```python
from build123d import *

# Parameters (mm, degrees)
SKETCH_1_W          = 12
SKETCH_1_H          = 10
EXTRUDE_1_DEPTH     = 0.8
CUT_EXTRUDE_1_REACH = 9.851
SKETCH_2_R          = 1.5
SKETCH_2_R_2        = 0.75
SKETCH_2_R_3        = 0.375
FILLET_1_R          = 1
SKETCH_5_R          = 0.5
CUT_EXTRUDE_2_DEPTH = 8.851114571
EXTRUDE_START       = 1
SKETCH_14_R         = 2
SKETCH_14_R_2       = 1.5
EXTRUDE_2_DEPTH     = 1


with BuildPart() as part:
    # Эскиз1 → Бобышка-Вытянуть1 (new body)
    with BuildSketch(Plane.XY):
        Rectangle(SKETCH_1_W, SKETCH_1_H)
    extrude(amount=EXTRUDE_1_DEPTH)

    # Эскиз2 → Вырез-Вытянуть1 (cut, up to next)
    with BuildSketch(Plane.XY.offset(0.8), mode=Mode.PRIVATE) as cut_extrude_1_sk1:
        Circle(SKETCH_2_R)
    cut_extrude_1_tool1 = extrude(cut_extrude_1_sk1.sketch, amount=-CUT_EXTRUDE_1_REACH, mode=Mode.PRIVATE) & part.part
    # Эскиз2 → Вырез-Вытянуть1 (cut, up to next)
    with BuildSketch(Plane.XY.offset(0.8), mode=Mode.PRIVATE) as cut_extrude_1_sk2:
        with Locations((-3.6, -3)):
            Circle(SKETCH_2_R_2)
    cut_extrude_1_tool2 = extrude(cut_extrude_1_sk2.sketch, amount=-CUT_EXTRUDE_1_REACH, mode=Mode.PRIVATE) & part.part
    # Эскиз2 → Вырез-Вытянуть1 (cut, up to next)
    with BuildSketch(Plane.XY.offset(0.8), mode=Mode.PRIVATE) as cut_extrude_1_sk3:
        with Locations((3.6, 3)):
            Circle(SKETCH_2_R_2)
    cut_extrude_1_tool3 = extrude(cut_extrude_1_sk3.sketch, amount=-CUT_EXTRUDE_1_REACH, mode=Mode.PRIVATE) & part.part
    # Эскиз2 → Вырез-Вытянуть1 (cut, up to next)
    with BuildSketch(Plane.XY.offset(0.8), mode=Mode.PRIVATE) as cut_extrude_1_sk4:
        with Locations((3.25, -2)):
            Circle(SKETCH_2_R_3)
    cut_extrude_1_tool4 = extrude(cut_extrude_1_sk4.sketch, amount=-CUT_EXTRUDE_1_REACH, mode=Mode.PRIVATE) & part.part
    # Эскиз2 → Вырез-Вытянуть1 (cut, up to next)
    with BuildSketch(Plane.XY.offset(0.8), mode=Mode.PRIVATE) as cut_extrude_1_sk5:
        with Locations((-3.25, 2)):
            Circle(SKETCH_2_R_3)
    cut_extrude_1_tool5 = extrude(cut_extrude_1_sk5.sketch, amount=-CUT_EXTRUDE_1_REACH, mode=Mode.PRIVATE) & part.part
    add(cut_extrude_1_tool1.solids().sort_by_distance((0, 0, 0.8))[0], mode=Mode.SUBTRACT)
    add(cut_extrude_1_tool2.solids().sort_by_distance((-3.6, -3, 0.8))[0], mode=Mode.SUBTRACT)
    add(cut_extrude_1_tool3.solids().sort_by_distance((3.6, 3, 0.8))[0], mode=Mode.SUBTRACT)
    add(cut_extrude_1_tool4.solids().sort_by_distance((3.25, -2, 0.8))[0], mode=Mode.SUBTRACT)
    add(cut_extrude_1_tool5.solids().sort_by_distance((-3.25, 2, 0.8))[0], mode=Mode.SUBTRACT)

    # Скругление1
    fillet_1_edges = [part.edges().sort_by_distance(p)[0] for p in [
        (6, -5, 0.4),
        (-6, -5, 0.4),
        (-6, 5, 0.4),
        (6, 5, 0.4),
    ]]
    fillet(fillet_1_edges, radius=FILLET_1_R)

    # Эскиз5 → Вырез-Вытянуть2 (cut, through all)
    with BuildSketch(Plane.XY.offset(0.8)):
        with Locations((5, 0)):
            Circle(SKETCH_5_R)
        with Locations((-5, 0)):
            Circle(SKETCH_5_R)
    extrude(amount=-CUT_EXTRUDE_2_DEPTH, mode=Mode.SUBTRACT)

    # Эскиз14 → Бобышка-Вытянуть2 (add)
    with BuildSketch(Plane.XY.offset(0.8).offset(EXTRUDE_START)):
        with Locations(Location((0, 0, 0), (0, 0, 180))):
            Circle(SKETCH_14_R)
        Circle(SKETCH_14_R_2, mode=Mode.SUBTRACT)
    extrude(amount=-EXTRUDE_2_DEPTH)


solid = part.part
```
The model under review builds one solid part; all positions refer to its coordinate system, in mm. A direction names the side the tool comes from. Give positions to 0.01 mm unless a question says otherwise; leave off trailing zeros. Write each loop counter-clockwise with the first axis right and the second up, starting at its lowest first coordinate (ties: lowest second). Pieces come first, ordered by that corner, then holes. Notation, with made-up numbers: (-34.75, 9.25) -> (22.25, 9.25) arc R21 ccw to (22.25, 35.25) -> close; hole circle Ø3 at (16, 75.5). An arc over 180 degrees is marked (long way). Answer in a Markdown table with one row per item.
1) Add section C-C on z = 0.5. State the section outline as (x, y) points (3 decimals).
Worked answers:
| item | result |
|---|---|
| outline | (-6, -4) arc R1 ccw to (-5, -5) -> (5, -5) arc R1 ccw to (6, -4) -> (6, 4) arc R1 ccw to (5, 5) -> (-5, 5) arc R1 ccw to (-6, 4) -> close; hole circle Ø1 at (-5, 0); hole circle Ø1.5 at (-3.6, -3); hole circle Ø0.75 at (-3.25, 2); hole circle Ø3 at (0, 0); hole circle Ø1.5 at (3.6, 3); hole circle Ø0.75 at (3.25, -2); hole circle Ø1 at (5, 0) |
2) Clearance check with a flat-ended pin moving along its axis: P1, Ø0.9, axis at x = -3.6, y = -3, coming from the +Z side. State where the tip first meets the part, or that it passes through.
Worked answers:
| item | result |
|---|---|
| P1 | through |
3) Add section B-B on y = 3. State the section outline as (x, z) points.
Worked answers:
| item | result |
|---|---|
| outline | (-6, 0) -> (2.85, 0) -> (2.85, 0.8) -> (-6, 0.8) -> close; (4.35, 0) -> (6, 0) -> (6, 0.8) -> (4.35, 0.8) -> close |
4) Add section D-D on y = 0.25. State the section outline as (x, z) points, plus the area to 3 significant figures.
Worked answers:
| item | result |
|---|---|
| outline | (-6, 0) -> (-5.43, 0) -> (-5.43, 0.8) -> (-6, 0.8) -> close; (-4.57, 0) -> (-1.48, 0) -> (-1.48, 1.8) -> (-1.98, 1.8) -> (-1.98, 0.8) -> (-4.57, 0.8) -> close; (1.48, 0) -> (4.57, 0) -> (4.57, 0.8) -> (1.98, 0.8) -> (1.98, 1.8) -> (1.48, 1.8) -> close; (5.43, 0) -> (6, 0) -> (6, 0.8) -> (5.43, 0.8) -> close |
| area | 6.86 mm² |
5) For L1, parallel to Y at x = 0, z = 0.85; L2, parallel to Z at x = -3, y = -2.25; L3, parallel to Y at x = -3.25, z = 0.5 (3 decimals), list the stretches that pass through material, from the lowest coordinate up. Write a range as [from, to].
Worked answers:
| item | result |
|---|---|
| L1 | [-2, -1.5], [1.5, 2] |
| L2 | [0, 0.8] |
| L3 | [-5, -3.663], [-2.337, 1.625], [2.375, 5] |
6) Tool access review of faces 4 (the cylindrical face through (0, 2, 1)), 5 (the cylindrical face through (-5.715, -4.699, 0.406)): name each direction out of +Z, -Z, +X, -X, +Y, -Y from which nothing blocks a thin tool from reaching the whole face with its end or side.
Worked answers:
| item | result |
|---|---|
| face 4 | +Z |
| face 5 | +Z, -Z, -X, -Y |
7) Add section A-A on x = 0. State the section outline as (y, z) points, plus the area to 3 significant figures.
Worked answers:
| item | result |
|---|---|
| outline | (-5, 0) -> (-1.5, 0) -> (-1.5, 1.8) -> (-2, 1.8) -> (-2, 0.8) -> (-5, 0.8) -> close; (1.5, 0) -> (5, 0) -> (5, 0.8) -> (2, 0.8) -> (2, 1.8) -> (1.5, 1.8) -> close |
| area | 6.60 mm² |
8) Mouldability with a two-part tool opening along Y and no side actions: class faces 1 (the flat face through (-0.1, 2.3, 0.8)), 2 (the cylindrical face through (2.85, 3.03, 0.41)), 3 (the cylindrical face through (-5.715, 4.699, 0.406)) as +Y half, -Y half, draft (parallel to the pull), parting line (faces both ways), or undercut.
Worked answers:
| item | result |
|---|---|
| face 1 | draft |
| face 2 | undercut |
| face 3 | +Y half |
